Can you work these out from the model? Positions are in its coordinate system, mm. A direction names the side the tool comes from. Give positions to 0.01 mm unless a question says otherwise; leave off trailing zeros. Loops run counter-clockwise (first coordinate to the right, second up) from the corner with the lowest first, then second, coordinate; pieces in that order, holes last.
from build123d import *

# Parameters (mm, degrees)
F0_W     = 1800
F0_H     = 500
F1_DEPTH = 600
F2_W     = 1780
F2_H     = 480
F3_DEPTH = 590
F5_W     = 150
F5_H     = 10
F5_W_2   = 300
F7_DEPTH = 500
F6_W     = 240
F6_H     = 480
F6_W_2   = 400
F6_H_2   = 474.8058223724
F8_DEPTH = 10


with BuildPart() as f1:
    # F0 (on Front) → F1 (new body)
    with BuildSketch(Plane.XZ):
        Rectangle(F0_W, F0_H)
    extrude(amount=F1_DEPTH)

    # F2 (on face) → F3 (cut)
    with BuildSketch(Plane.XZ.offset(600)):
        Rectangle(F2_W, F2_H)
    extrude(amount=-F3_DEPTH, mode=Mode.SUBTRACT)

    # F5 (on face) → F7 (join)
    with BuildSketch(Plane(origin=(0, 0, -250), x_dir=(1, 0, 0), z_dir=(0, 0, -1))):
        with Locations((525, 605)):
            Rectangle(F5_W, F5_H)
        with Locations((0, 605)):
            Rectangle(F5_W_2, F5_H)
        with Locations((-525, 605)):
            Rectangle(F5_W, F5_H)
    extrude(amount=-F7_DEPTH)

    # F6 (on face) → F8 (join)
    with BuildSketch(Plane.XZ.offset(10)):
        with Locations((-770, 0)):
            Rectangle(F6_W, F6_H)
        with Locations((150, 0)):
            Rectangle(F6_W_2, F6_H)
        with Locations((770, 2.5970888138)):
            Rectangle(F6_W, F6_H_2)
    extrude(amount=F8_DEPTH)


solid = f1.part
(1) Suppose I cut it at B-B on z = 147. List the corners of the cut face in (x, y) for me, plus the area to 3 significant figures.
Returned:
outline: (-900, -600) - (-890, -600) - (-890, -20) - (-650, -20) - (-650, -10) - (-50, -10) - (-50, -20) - (350, -20) - (350, -10) - (650, -10) - (650, -20) - (890, -20) - (890, -600) - (900, -600) - (900, 0) - (-900, 0) - close; (-600, -610) - (-450, -610) - (-450, -600) - (-600, -600) - close; (-150, -610) - (150, -610) - (150, -600) - (-150, -600) - close; (450, -610) - (600, -610) - (600, -600) - (450, -600) - close
area: 44,600 mm2
(2) Suppose I cut it at A-A on x = 516. List the corners of the cut face in (y, z) for me.
Returned:
outline: (-610, -250) - (0, -250) - (0, 250) - (-610, 250) - close; hole (-600, -240) - (-10, -240) - (-10, 240) - (-600, 240) - close
(3) Will these pins go through, and if not, where does the flat tip stop? P1, Ø8, axis at x = -363, z = -243.5, coming from the -Y side; P2, Ø3, axis at y = -607, z = 81.5, coming from the +X side; P3, Ø5, axis at y = -604.5, z = -10, coming from the -X side.
Returned:
P1: stops at y = -600
P2: stops at x = 600
P3: stops at x = -600
(4) Thinking about a two-plate mould opening in X: for faces 5 (the flat face through (-900, -296, -3)), 6 (the flat face through (496, -10, 3)), 7 (the flat face through (-13, -309, 250)), which applies, pulls with the +X half, pulls with the -X half, needs draft (parallel to the pull), parting line crosses it, or undercut?
Returned:
face 5: pulls with the -X half
face 6: undercut
face 7: needs draft
(5) Suppose I cut it at C-C on y = -133. List the corners of the cut face in (x, z) for me.
Returned:
outline: (-900, -250) - (900, -250) - (900, 250) - (-900, 250) - close; hole (-890, -240) - (890, -240) - (890, 240) - (-890, 240) - close
(6) Which directions (+Z, -Z, +X, -X, +Y, -Y) give clear straight access to the entire face, cutting with the end or side of a thin tool? Please do faces 1 (the flat face through (-890, -314, -3)), 2 (the flat face through (-2, -600, -3)), 3 (the flat face through (894, -600, 112)), 4 (the flat face through (900, -296, -3)).
Returned:
face 1: -Y
face 2: none
face 3: +Z, -Z, +X, -Y
face 4: +Z, -Z, +X, +Y, -Y
(7) Suppose I cut it at D-D on x = 222. List the corners of the cut face in (y, z) for me, plus the area to 3 significant figures.
Returned:
outline: (-600, -250) - (0, -250) - (0, 250) - (-600, 250) - (-600, 240) - (-20, 240) - (-20, -240) - (-600, -240) - close
area: 21,600 mm2
(8) Please list where these lines run through material, in increasing order: probe 1 along Z at (x, y) = (-311, -537.5); probe 2 along X at (y, z) = (-375, 207); probe 3 along Y at (x, z) = (497, 23.5).
Returned:
probe 1: z = -250 to -240, 240 to 250
probe 2: x = -900 to -890, 890 to 900
probe 3: y = -610 to -600, -10 to 0
